```python
from build123d import *

# Parameters (mm, degrees)
CUT_EXTRUDE1_DEPTH      = 63.771171727
CUT_EXTRUDE1_DEPTH_BACK = 63.771171727
SKETCH6_R               = 3.25


with BuildPart() as part:
    # Sweep1: sweep along a path in Sketch1
    with BuildLine(Plane(origin=(0, 0, 0), x_dir=(1, 0, 0), z_dir=(0, 1, 0))) as sweep1_path:
        CenterArc((0, 0), 38.1, 0, 360)
    # Sketch2 → Sweep1 (sweep)
    with BuildSketch(Plane(origin=(0, 0, 0), x_dir=(0, 0, -1), z_dir=(1, 0, 0))):
        Polygon((-38.1, 5), (-43.1, 10), (-43.1, 5.5), (-40.1, 2.5), (-40.1, -2.5), (-43.1, -5.5), (-43.1, -10), (-38.1, -5), (0, -5), (0, 0), (0, 5), align=None)
    sweep(path=sweep1_path.line)

    # Sketch6 → Cut-Extrude1 (cut, two sides: drawn at the far end of the back side and taken through both)
    with BuildSketch(Plane(origin=(0, -5, 0), x_dir=(-1, 0, 0), z_dir=(0, -1, 0)).offset(-CUT_EXTRUDE1_DEPTH_BACK)):
        with Locations(Location((0, 0, 0), (0, 0, 270))):
            Circle(SKETCH6_R)
    extrude(amount=CUT_EXTRUDE1_DEPTH + CUT_EXTRUDE1_DEPTH_BACK, mode=Mode.SUBTRACT)


solid = part.part
```
Read the model definition and answer for the solid it produces. Units are mm, in the model's axes. A direction names the side the tool comes from. Give positions to 0.01 mm unless a question says otherwise; leave off trailing zeros. Order: outer loops, then holes, each group sorted by start corner. A loop starts at its lowest first (then second) coordinate and runs counter-clockwise, first axis right, second up.
(1) Straight lines are drawn through the part: L1, parallel to Y at x = -30, z = -13; L2, parallel to Y at x = -38, z = 17.5; L3, parallel to X at y = -5.25, z = -18.5. For each, find the intervals that lie inside material, in ascending order.
(2) Find section A-A (y = 8.75). Give the vertices of the cut face in (x, z).
(3) For a pull along Y with two mould halves and no side action, classify faces 1 (the cylindrical face through (37.04, -0.04, 15.36)), 2 (the conical face through (-8.31, -5.24, 37.43)), 3 (the cylindrical face through (19.888, -7.781, 38.237)) as released by +Y, released by -Y, zero draft, split by the parting line, or undercut.
(4) For faces 4 (the conical face through (-8.724, 2.646, 39.289)), 5 (the cylindrical face through (19.888, 7.719, 38.237)), determine the directions among +Z, -Z, +X, -X, +Y, -Y from which every point of the face is accessible in a straight line to the end or side of a thin tool.
(5) Find section B-B (y = 4). Give the vertices of the cut face in (x, z).
(6) Given pin 1 (2 mm diameter, centred on x = 24.5, y = -5.5, fed in from -Z); pin 2 (5 mm diameter, centred on x = 0.5, y = -1, fed in from -Z); pin 3 (12 mm diameter, centred on x = 16, y = 3.5, fed in from -Z), each flat-ended and moving along its own axis, determine where each tip first touches the part or whether it passes through.
Result sheet:
1. L1: y = -5 to 5
1. L2: y = -8.74 to -4.24, 4.24 to 8.74
1. L3: x = -38.65 to -33.59, 33.59 to 38.65
2. outline: circle Ø86.2 at (0, 0); hole circle Ø83.7 at (0, 0)
3. face 1: undercut
3. face 2: released by -Y
3. face 3: zero draft
4. face 4: none
4. face 5: +Y, -Y
5. outline: circle Ø83.2 at (0, 0); hole circle Ø6.5 at (0, 0)
6. pin 1: stops at z = -36.13
6. pin 2: stops at z = -41.1
6. pin 3: stops at z = -41.84
